```python
from build123d import *

# Parameters (mm, degrees)
F0_W           = 25.5
F0_H           = 10
F1_DEPTH       = 15
F2_D           = 3.4
F3_W           = 10
F3_H           = 7
F4_DEPTH       = 2.5
F5_W           = 10
F5_H           = 10
F6_DEPTH       = 5
F8_D           = 4.5
F8_CSINK_D     = 8.96
F8_CSINK_ANGLE = 90
F9_SIZE        = 2
F11_DEPTH      = 2.5


with BuildPart() as f1:
    # F0 (on Top) → F1 (new body)
    with BuildSketch(Plane.XY):
        Rectangle(F0_W, F0_H)
    extrude(amount=-F1_DEPTH)

    # F2 (through all)
    with Locations(Plane.XY):
        with Locations((-9.55, 0), (9.45, 0)):
            Hole(F2_D / 2)

    # F3 (on face) → F4 (cut)
    with BuildSketch(Plane.XY):
        with Locations((-0.05, 0)):
            Rectangle(F3_W, F3_H)
    extrude(amount=-F4_DEPTH, mode=Mode.SUBTRACT)

    # F5 (on face) → F6 (join)
    with BuildSketch(Plane(origin=(0, 0, -15), x_dir=(1, 0, 0), z_dir=(0, 0, -1))):
        with Locations((0, 10)):
            Rectangle(F5_W, F5_H)
        with Locations((0, -10)):
            Rectangle(F5_W, F5_H)
    extrude(amount=-F6_DEPTH)

    # F8 (through all)
    with Locations(Plane.XY.offset(-10)):
        with Locations((0, -10), (0, 10)):
            CounterSinkHole(F8_D / 2, F8_CSINK_D / 2, counter_sink_angle=F8_CSINK_ANGLE)

    # F9
    f9_edges = [f1.edges().sort_by_distance(p)[0] for p in [
        (-5, 15, -12.5),
        (5, 15, -12.5),
        (5, 5, -12.5),
        (-5, 5, -12.5),
        (5, -5, -12.5),
        (5, -15, -12.5),
        (-5, -15, -12.5),
    ]]
    chamfer(f9_edges, length=F9_SIZE)

    # F10 (on face) → F11 (cut)
    with BuildSketch(Plane(origin=(0, 0, -15), x_dir=(1, 0, 0), z_dir=(0, 0, -1))):
        Polygon((6.7653212483, -1.55), (9.45, -3.1), (12.1346787517, -1.55), (12.1346787517, 1.55), (9.45, 3.1), (6.7653212483, 1.55), align=None)
        Polygon((-12.1346787517, -1.55), (-9.45, -3.1), (-6.7653212483, -1.55), (-6.7653212483, 1.55), (-9.45, 3.1), (-12.1346787517, 1.55), align=None)
    extrude(amount=-F11_DEPTH, mode=Mode.SUBTRACT)


solid = f1.part
```
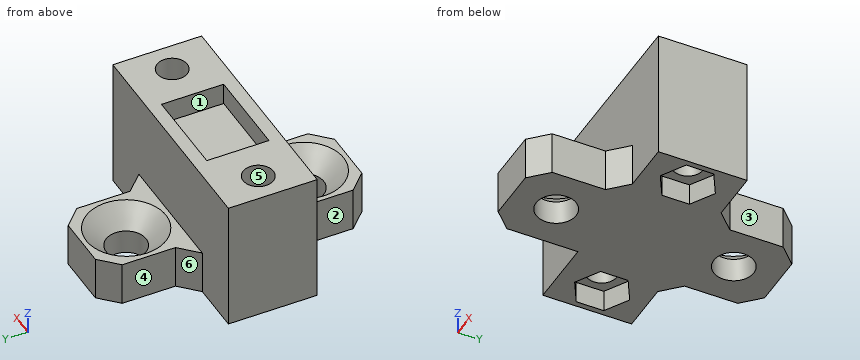
Part model, mm, in its own coordinate system. Face numbers are marked on the shaded views. A direction names the side the tool comes from. Give positions to 0.01 mm unless a question says otherwise; leave off trailing zeros. Order: outer loops, then holes, each group sorted by start corner. A loop starts at its lowest first (then second) coordinate and runs counter-clockwise, first axis right, second up. Notation, with made-up numbers: M 67,69 L 106,69 A19 ccw 106,105 Z; hole C 0,5 d6. An arc over 180 degrees is marked long. Use a Markdown table: item, result. Add a question column.
(1) Saw through at C-C, the plane z = -6. Give the cut face in (x, y), and give its area (3 significant figures).
(2) Saw through at A-A, the plane y = 0. Give the cut face in (x, z).
(3) 3-axis set-ups, long thin cutter, end or side, ignore diameter. For the marked faces 1, 2 and 3: which of +Z, -Z, +X, -X, +Y, -Y reach the whole face in a straight line?
(4) Saw through at D-D, the plane y = 10. Give the cut face in (x, z), and give its area (3 significant figures).
(5) Mould opens along Y. For the marked faces 4, 5 and 6 say: +Y half, -Y half, draft (parallel to the pull), parting line (faces both ways), or undercut.
(6) Probe line 1 along Y through (x, z) = (0, -13.45); line 2 along X through (y, z) = (-10, -14.1); line 3 along X through (y, z) = (0.5, -2.25). List the from-to ranges inside material, lowest first. Write a range as [from, to].
(7) Saw through at B-B, the plane x = 0. Give the cut face in (y, z).
(8) Drop flat-ended pins along their axis: P1, Ø2, axis at x = -2, y = 1, coming from the +Z side; P2, Ø1.5, axis at y = -10.5, z = -13.5, coming from the +X side; P3, Ø5, axis at x = 7.5, z = -9, coming from the +Y side. Give the stop position or say it passes through.
Answer key:
| question | item | result |
|---|---|---|
| 1 | outline | M -12.75,-5 L 12.75,-5 L 12.75,5 L -12.75,5 Z; hole C -9.55,0 d3.4; hole C 9.45,0 d3.4 |
| 1 | area | 237 mm^2 |
| 2 | outline | M -12.75,-15 L -12.13,-15 L -12.13,-12.5 L -11.25,-12.5 L -11.25,0 L -12.75,0 Z; M -7.85,-12.5 L -6.77,-12.5 L -6.77,-15 L 6.77,-15 L 6.77,-12.5 L 7.75,-12.5 L 7.75,0 L 4.95,0 L 4.95,-2.5 L -5.05,-2.5 L -5.05,0 L -7.85,0 Z; M 11.15,-12.5 L 12.13,-12.5 L 12.13,-15 L 12.75,-15 L 12.75,0 L 11.15,0 Z |
| 3 | face 1 | +Z |
| 3 | face 2 | +Z, -Z, -X, -Y |
| 3 | face 3 | +Z, -Z, +X, +Y |
| 4 | outline | M -5,-15 L -2.25,-15 L -2.25,-12.23 L -4.48,-10 L -5,-10 Z; M 2.25,-15 L 5,-15 L 5,-10 L 4.48,-10 L 2.25,-12.23 Z |
| 4 | area | 22.5 mm^2 |
| 5 | face 4 | draft |
| 5 | face 5 | undercut |
| 5 | face 6 | +Y half |
| 6 | line 1 | [-15, -12.25], [-7.75, 7.75], [12.25, 15] |
| 6 | line 2 | [-5, -2.25], [2.25, 5] |
| 6 | line 3 | [-12.75, -11.17], [-7.93, -5.05], [4.95, 7.83], [11.07, 12.75] |
| 7 | outline | M -15,-15 L -12.25,-15 L -12.25,-12.23 L -14.48,-10 L -15,-10 Z; M -7.75,-15 L 7.75,-15 L 7.75,-12.23 L 5.52,-10 L 5,-10 L 5,0 L 3.5,0 L 3.5,-2.5 L -3.5,-2.5 L -3.5,0 L -5,0 L -5,-10 L -5.52,-10 L -7.75,-12.23 Z; M 12.25,-15 L 15,-15 L 15,-10 L 14.48,-10 L 12.25,-12.23 Z |
| 8 | P1 | z = -2.5 |
| 8 | P2 | x = 5 |
| 8 | P3 | y = 6.79 |
